Verification items for the finished model (mm, model axes). A direction names the side the tool comes from. Coordinates: 2 decimals unless noted, no trailing zeros. Order: outer loops, then holes, each group sorted by start corner. A loop starts at its lowest first (then second) coordinate and runs counter-clockwise, first axis right, second up.
Q1. Cross-section at B-B, the plane z = 35. Record the boundary of the cut face in (x, y).
Q2. Set-up check for faces 1 (the cylindrical face through (0, 24, 2)), 2 (the cylindrical face through (20.07, -2.71, 12.797)): record each of +Z, -Z, +X, -X, +Y, -Y from which the full face is reachable in a straight line by a thin tool's end or side.
Q3. Cross-section at C-C, the plane x = 21. Record the boundary of the cut face in (y, z).
Q4. Cross-section at A-A, the plane y = 0. Record the boundary of the cut face in (x, z).
Q5. Thickness scan on line 1 (X direction, y = -1, z = 26); line 2 (Z direction, x = 20.25, y = 0); line 3 (Y direction, x = 16, z = 22). Record the ranges inside material, lowest first.
Q6. Depth check by flat-ended pin: P1, Ø10, axis at y = 4.5, z = 20.5, coming from the +X side. Enter the tip coordinate at first touch or a pass-through.
from build123d import *

# Parameters (mm, degrees)
F0_W     = 50
F0_H     = 50
F1_DEPTH = 50
F2_R     = 12.5
F3_DEPTH = 10
F4_R     = 5


with BuildPart() as f1:
    # F0 (on Top) → F1 (new body)
    with BuildSketch(Plane.XY):
        Rectangle(F0_W, F0_H)
    extrude(amount=F1_DEPTH)

    # F2 (on face) → F3 (cut)
    with BuildSketch(Plane.YZ.offset(25)):
        with Locations((0, 25)):
            Circle(F2_R)
    extrude(amount=-F3_DEPTH, mode=Mode.SUBTRACT)

    # F4
    f4_edges = [f1.edges().sort_by_distance(p)[0] for p in [
        (25, 0, 0),
        (25, 25, 25),
        (25, 0, 50),
        (25, -25, 25),
        (0, 25, 0),
        (0, -25, 0),
        (0, -25, 50),
        (0, 25, 50),
        (-25, 25, 25),
        (-25, 0, 0),
        (-25, 0, 50),
        (-25, -25, 25),
    ]]
    fillet(f4_edges, radius=F4_R)


solid = f1.part
Check values:
1. outline: (-25, -20) arc R5 ccw to (-20, -25) - (20, -25) arc R5 ccw to (25, -20) - (25, -7.5) - (15, -7.5) - (15, 7.5) - (25, 7.5) - (25, 20) arc R5 ccw to (20, 25) - (-20, 25) arc R5 ccw to (-25, 20) - close
2. face 1: -Z, +X, -X, +Y
2. face 2: +X
3. outline: (-24.9, 5) arc R4.9 ccw to (-20, 0.1) - (20, 0.1) arc R4.9 ccw to (24.9, 5) - (24.9, 45) arc R4.9 ccw to (20, 49.9) - (-20, 49.9) arc R4.9 ccw to (-24.9, 45) - close; hole circle Ø25 at (0, 25)
4. outline: (-25, 5) arc R5 ccw to (-20, 0) - (20, 0) arc R5 ccw to (25, 5) - (25, 12.5) - (15, 12.5) - (15, 37.5) - (25, 37.5) - (25, 45) arc R5 ccw to (20, 50) - (-20, 50) arc R5 ccw to (-25, 45) - close
5. line 1: x = -25 to 15
5. line 2: z = 0.01 to 12.5, 37.5 to 49.99
5. line 3: y = -25 to -12.13, 12.13 to 25
6. P1: stops at x = 15
